from build123d import *

# Parameters (mm, degrees)
SKETCH_1_W          = 52
SKETCH_1_H          = 25
EXTRUDE_1_DEPTH     = 3
SKETCH_2_W          = 3
SKETCH_2_H          = 25
EXTRUDE_2_DEPTH     = 50
CUT_EXTRUDE_1_DEPTH = 76.294422104


with BuildPart() as part:
    # 스케치1 → 보스-돌출1 (new body)
    with BuildSketch(Plane.XY):
        Rectangle(SKETCH_1_W, SKETCH_1_H)
    extrude(amount=EXTRUDE_1_DEPTH)

    # 스케치2 → 보스-돌출2 (add)
    with BuildSketch(Plane.XY.offset(3)):
        with Locations((-24.5, 0)):
            Rectangle(SKETCH_2_W, SKETCH_2_H)
        with Locations((24.5, 0)):
            Rectangle(SKETCH_2_W, SKETCH_2_H)
    extrude(amount=EXTRUDE_2_DEPTH)

    # 스케치3 → 컷-돌출1 (cut, through all)
    with BuildSketch(Plane(origin=(26, 0, 0), x_dir=(0, 0, -1), z_dir=(1, 0, 0))):
        with BuildLine():
            ThreePointArc((-53, 1.56e-07), (-49.33883471, 8.83883482), (-40.5, 12.5))
            Line((-40.5, 12.5), (-53, 12.5))
            Line((-53, 12.5), (-53, 1.56e-07))
        make_face()
        with BuildLine():
            Line((-53, -12.5), (-40.5, -12.5))
            ThreePointArc((-40.5, -12.5), (-49.33883482, -8.83883471), (-53, 1.56e-07))
            Line((-53, 1.56e-07), (-53, -12.5))
        make_face()
    extrude(amount=-CUT_EXTRUDE_1_DEPTH, mode=Mode.SUBTRACT)


solid = part.part
CAD build for the part. Positions are in the model's coordinates, mm. A direction names the side the tool comes from. Give positions to 0.01 mm unless a question says otherwise; leave off trailing zeros. Order: outer loops, then holes, each group sorted by start corner. A loop starts at its lowest first (then second) coordinate and runs counter-clockwise, first axis right, second up. Notation, with made-up numbers: (-16.5, 6) -> (4.5, 6) arc R14 cw to (4.5, 24) -> close; hole circle Ø2 at (-16, 63). An arc over 180 degrees is marked (long way). Return JSON: item names as keys, results as strings.
Q1. Saw through at C-C (z = 45). Write the cut outline in (x, y), then the cut area to 3 significant figures.
Working result:
{"outline": "(-26, -11.66) -> (-23, -11.66) -> (-23, 11.66) -> (-26, 11.66) -> close; (23, -11.66) -> (26, -11.66) -> (26, 11.66) -> (23, 11.66) -> close", "area": "140 mm²"}
Q2. Mould opens along X. For faces 3 (the face through (0, 0, 0)), 4 (the face through (26, 0, 26)), 5 (the face through (23, 0, 28)) say: pulls with the +X half, pulls with the -X half, needs draft (parallel to the pull), parting line crosses it, or undercut.
Working result:
{"face 3": "needs draft", "face 4": "pulls with the +X half", "face 5": "undercut"}
Q3. Drill centre lines: line 1 (X direction, y = -4, z = 41.5); line 2 (Z direction, x = -7, y = 1.5). Where is each one in solid material? Low to high.
Working result:
{"line 1": "-26 to -23, 23 to 26", "line 2": "0 to 3"}
Q4. Which spindle directions (+Z, -Z, +X, -X, +Y, -Y) get a long thin tool onto all of the face, cutting with end or side? Do faces 1 (the face through (-26, 0, 26)), 2 (the face through (-23, 0, 28)). Say none if no direction does.
Working result:
{"face 1": "+Z, -Z, -X, +Y, -Y", "face 2": "+Z, +Y, -Y"}
Q5. Flat gauge pins, fed straight in: pin 1 (3 mm diameter, centred on x = 9, y = 0.5, fed in from -Z); pin 2 (12 mm diameter, centred on x = 8.5, y = -9, fed in from +Z). Where does each tip first touch, or does it go through?
Working result:
{"pin 1": "z = 0", "pin 2": "z = 3"}
Q6. Saw through at B-B (y = 4.25). Write the cut outline in (x, z), then the cut area to 3 significant figures.
Working result:
{"outline": "(-26, 0) -> (26, 0) -> (26, 52.26) -> (23, 52.26) -> (23, 3) -> (-23, 3) -> (-23, 52.26) -> (-26, 52.26) -> close", "area": "452 mm²"}
Q7. Saw through at D-D (x = -13). Write the cut outline in (y, z), then the cut area to 3 significant figures.
Working result:
{"outline": "(-12.5, 0) -> (12.5, 0) -> (12.5, 3) -> (-12.5, 3) -> close", "area": "75.0 mm²"}
Q8. Saw through at A-A (z = 32.5). Write the cut outline in (x, y).
Working result:
{"outline": "(-26, -12.5) -> (-23, -12.5) -> (-23, 12.5) -> (-26, 12.5) -> close; (23, -12.5) -> (26, -12.5) -> (26, 12.5) -> (23, 12.5) -> close"}
